```python
from build123d import *

# Parameters (mm, degrees)
BOSS_EXTRU_1_DEPTH            = 729
ENL_V_MAT_EXTRU_1_DEPTH       = 727
ESQUISSE3_W                   = 40
ESQUISSE3_H                   = 40
BOSS_EXTRU_2_DEPTH            = 814.58026
ENL_V_MAT_EXTRU_2_DEPTH       = 829.69546376
ENL_V_MAT_EXTRU_2_DEPTH_BACK  = 829.69546376
ESQUISSE4_W                   = 98.578400591
ESQUISSE4_H                   = 147.950096535
ESQUISSE4_W_2                 = 77.840885054
ESQUISSE4_H_2                 = 46.084081252
ESQUISSE7_W                   = 821.544509843
ESQUISSE7_H                   = 616.158382383
ESQUISSE7_W_2                 = 40
ESQUISSE7_H_2                 = 40
ENL_V_MAT_EXTRU_6_DEPTH       = 828.213294061
ESQUISSE8_W                   = 32
ESQUISSE8_H                   = 32
ENL_V_MAT_EXTRU_9_DEPTH       = 828.213294061
CONG_2_R                      = 2
ENL_V_MAT_EXTRU_10_DEPTH      = 815.022307134
ENL_V_MAT_EXTRU_10_DEPTH_BACK = 815.022307134
ESQUISSE9_W                   = 398.467294392
ESQUISSE9_H                   = 786.430421472


with BuildPart() as part:
    # Esquisse1 → Boss.-Extru.1 (new body)
    with BuildSketch(Plane.XY):
        Polygon((0, 0), (258, 0), (0, 256), align=None)
    extrude(amount=BOSS_EXTRU_1_DEPTH)

    # Esquisse2 → Enlèv. mat.-Extru.1 (cut)
    with BuildSketch(Plane.ZY):
        Polygon((0, 256), (729, 0), (729, 256), align=None)
    extrude(amount=-ENL_V_MAT_EXTRU_1_DEPTH, mode=Mode.SUBTRACT)

    # Esquisse3 → Boss.-Extru.2 (add)
    with BuildSketch(Plane(origin=(0, 256, 0), x_dir=(0.948516525956314, 0.10519863837129277, -0.2987467932423567), z_dir=(0.31672753768478995, -0.31427228545467534, 0.8949394378767902))):
        with Locations((20, -20)):
            Rectangle(ESQUISSE3_W, ESQUISSE3_H)
    extrude(amount=BOSS_EXTRU_2_DEPTH)

    # Esquisse4 → Enlèv. mat.-Extru.2 (cut, two sides: drawn at the far end of the back side and taken through both)
    with BuildSketch(Plane(origin=(0, 0, 0), x_dir=(-1, 0, 0), z_dir=(0, -1, 0)).offset(-ENL_V_MAT_EXTRU_2_DEPTH_BACK)):
        with Locations((-307.289200295, -655.024951733)):
            Rectangle(ESQUISSE4_W, ESQUISSE4_H)
        with Locations((-38.920442527, 23.042040626)):
            Rectangle(ESQUISSE4_W_2, ESQUISSE4_H_2)
    extrude(amount=ENL_V_MAT_EXTRU_2_DEPTH + ENL_V_MAT_EXTRU_2_DEPTH_BACK, mode=Mode.SUBTRACT)

    # Esquisse7 → Enlèv. mat.-Extru.6 (cut, through all)
    with BuildSketch(Plane(origin=(0, 256, 0), x_dir=(0.948516525956314, 0.10519863837129277, -0.2987467932423567), z_dir=(0.31672753768478995, -0.31427228545467534, 0.8949394378767902))):
        with Locations((22.907114777, -53.97111912)):
            Rectangle(ESQUISSE7_W, ESQUISSE7_H)
        with Locations((20, -20)):
            Rectangle(ESQUISSE7_W_2, ESQUISSE7_H_2, mode=Mode.SUBTRACT)
    extrude(amount=ENL_V_MAT_EXTRU_6_DEPTH, mode=Mode.SUBTRACT)

    # Esquisse8 → Enlèv. mat.-Extru.9 (cut, through all)
    with BuildSketch(Plane(origin=(0, 256, 0), x_dir=(0.948516525956314, 0.10519863837129277, -0.2987467932423567), z_dir=(0.31672753768478995, -0.31427228545467534, 0.8949394378767902))):
        with Locations((20, -20)):
            Rectangle(ESQUISSE8_W, ESQUISSE8_H)
    extrude(amount=ENL_V_MAT_EXTRU_9_DEPTH, mode=Mode.SUBTRACT)

    # Congé2
    cong_2_edges = [part.edges().sort_by_distance(p)[0] for p in [
        (131.343588352, 126.087109834, 357.878000354),
        (133.224361668, 94.037568496, 352.563722265),
        (150.092295167, 110.783988508, 304.90200319),
        (148.211521852, 142.833529846, 310.21628128),
        (129, 128, 364.5),
        (150.084916875, 148.933025015, 304.922851157),
        (152.435883519, 108.871098342, 298.280003544),
        (131.350966645, 87.938073327, 357.857152388),
    ]]
    fillet(cong_2_edges, radius=CONG_2_R)

    # Symétrie4: part across plane


with BuildPart() as part_1:
    add(part.part)
    add(part.part.mirror(Plane.XY))

    # Esquisse9 → Enlèv. mat.-Extru.10 (cut, two sides: drawn at the far end of the back side and taken through both)
    with BuildSketch(Plane(origin=(0, 0, 0), x_dir=(1, 0, 0), z_dir=(0, 1, 0)).offset(-ENL_V_MAT_EXTRU_10_DEPTH_BACK)):
        with Locations((201.342138883, -393.215210736)):
            Rectangle(ESQUISSE9_W, ESQUISSE9_H)
    extrude(amount=ENL_V_MAT_EXTRU_10_DEPTH + ENL_V_MAT_EXTRU_10_DEPTH_BACK, mode=Mode.SUBTRACT)


solid = part_1.part
```
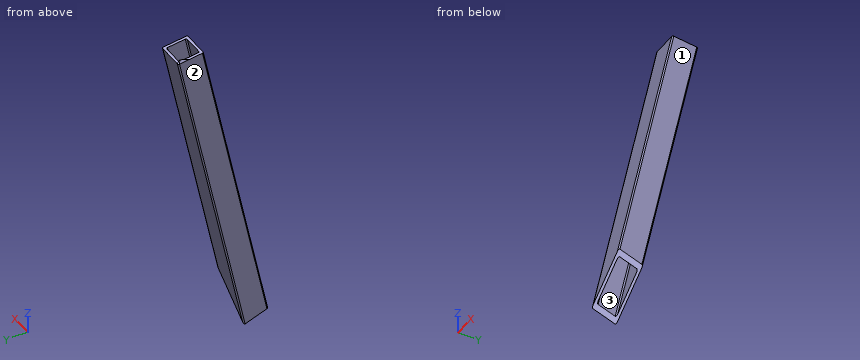
Check sheet for the modelled part. Datum: model origin and axes. Units: mm. Face numbers are marked on the shaded views. Round coordinates to 2 decimals unless told otherwise and drop trailing zeros. Write item = value, one per line. Start each with the question number.
Q1. Release check for a two-part mould opening along X. For the marked faces 1, 2 and 3 record: pulls with the +X half, pulls with the -X half, needs draft (parallel to the pull), parting line crosses it, or undercut.
Q2. Depth check by flat-ended pin: P1, Ø4.5, axis at y = 250, z = 1.5, coming from the +X side; P2, Ø1.5, axis at y = 42.5, z = -538, coming from the -X side. Enter the tip coordinate at first touch or a pass-through.
Q3. Thickness scan on L1, parallel to Y at x = 163, z = -393.5; L2, parallel to Y at x = 49.5, z = -55; L3, parallel to X at y = 197, z = -95.5. Record the ranges inside material, lowest first.
Derived:
q1.face_1 = pulls with the +X half
q1.face_2 = pulls with the -X half
q1.face_3 = undercut
q2.P1 = 43.12
q2.P2 = 192.88
q3.L1 = 75.43 to 79.67, 113.58 to 117.82
q3.L2 = 194.3 to 198.54, 232.45 to 236.69
q3.L3 = 36.62 to 40.84, 74.58 to 78.79
